Autodesk Inventor part; units mm, degrees
ref_plane "YZ Plane" through (0, 0, 0) normal (1, 0, 0) x (0, 1, 0)
ref_plane "XZ Plane" through (0, 0, 0) normal (0, 1, 0) x (-1, 0, 0)
ref_plane "XY Plane" through (0, 0, 0) normal (0, 0, 1) x (1, 0, 0)
sketch "Boceto1" plane through (0, 0, 0) normal (1, 0, 0) x (0, 1, 0)
  line L0 (0, 0) -> (0, -60)
  line L1 (0, -60) -> (10, -60)
  line L2 (10, -60) -> (10, -48)
  line L3 (10, -48) -> (35, -48)
  line L4 (35, -48) -> (35, -12)
  line L5 (35, -12) -> (10, -12)
  line L6 (10, -12) -> (10, 0)
  line L7 (10, 0) -> (0, 0)
  circle A0 centre (15, -30) radius 6
  dimension "d0" = 36
  dimension "d1" = 12
  dimension "d2" = 12
  dimension "d3" = 35
  dimension "d4" = 10
  dimension "d5" = 20
  dimension "d6" = 18
  dimension "d7" = 12
extrude "Extrusión1" add sketch "Boceto1" along normal blind 20
sketch "Boceto2" plane through (20, 0, 0) normal (1, 0, 0) x (0, 0, -1)
  circle A0 centre (30, 15) radius 6
  circle A1 centre (30, 15) radius 11
  point P0 (0, 0)
  dimension "d10" = 22
extrude "Extrusión2" cut sketch "Boceto2" against normal blind 7
sketch "Boceto3" plane through (0, 0, 0) normal (-1, 0, 0) x (0, 0, 1)
  circle A0 centre (-30, 15) radius 6
  circle A1 centre (-30, 15) radius 11
  point P0 (0, 0)
  dimension "d13" = 22
extrude "Extrusión3" cut sketch "Boceto3" against normal blind 7
sketch "Boceto4" plane through (0, 10, 0) normal (0, 1, 0) x (1, 0, 0)
  line L0 (20, 12) -> (20, 0)
  line L1 (0, 12) -> (0, 0)
  line L2 (20, 60) -> (20, 48)
  line L3 (0, 12) -> (20, 12)
  line L4 (0, 0) -> (20, 0)
  line L5 (0, 60) -> (20, 60)
  point P0 (10, 6)
  point P1 (10, 54)
  dimension "d16" = 20
  dimension "d17" = 10
  dimension "d18" = 10
  dimension "d19" = 12
  dimension "d20" = 6
  dimension "d21" = 6
hole "Agujero1" at (10, 10, -6) at (10, 10, -54) direction (0, -1, 0) diameter 5 end through all
fillet "Empalme1" radius 4 4 edges at (20, 5, 0) (20, 5, -60) (0, 5, -60) (0, 5, 0)
fillet "Empalme2" radius 2 2 edges at (10, 10, -12) (10, 10, -48)
fillet "Empalme3" radius 4 2 edges at (10, 35, -12) (10, 35, -48)
equation "\"d2\" = d1"
equation "\"d6\" = 0.5 * d0"
properties part number "Soporte_rueda_aluminio"
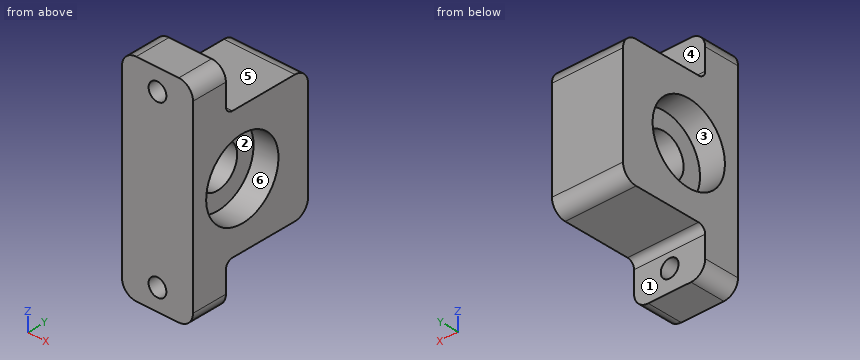
The model under review builds one solid part; all positions refer to its coordinate system, in mm. Face numbers are marked on the shaded views. A direction names the side the tool comes from. Give positions to 0.01 mm unless a question says otherwise; leave off trailing zeros. Write each loop counter-clockwise with the first axis right and the second up, starting at its lowest first coordinate (ties: lowest second). Pieces come first, ordered by that corner, then holes.
1. Wall thickness on L1, parallel to Z at x = 10, y = 3.5; L2, parallel to Z at x = 9.45, y = 15; L3, parallel to Y at x = 15.25, z = -30: over which ranges is each line inside the solid? List them lowest first.
2. Add section A-A, the plane x = 10. Write out the cut boundary in (y, z).
3. For P1, Ø11, axis at y = 14, z = -29, coming from the +X side; P2, Ø6, axis at x = 10, z = -54, coming from the +Y side; P3, Ø7, axis at y = 15, z = -30, coming from the +X side; P4, Ø8, axis at x = 11.5, y = 25, coming from the -Z side, all flat-tipped, find the tip position at first contact; note any pin that passes through.
4. Add section C-C, the plane y = 15. Write out the cut boundary in (x, z).
5. Draft analysis for pull direction Y (two halves, no side actions). For the marked faces 4, 5 and 6, state which applies: +Y half, -Y half, draft (parallel to the pull), parting line (faces both ways), or undercut.
6. Tool access review of the marked faces 1, 2 and 3: name each direction out of +Z, -Z, +X, -X, +Y, -Y from which nothing blocks a thin tool from reaching the whole face with its end or side.
7. Add section D-D, the plane x = 14.25. Write out the cut boundary in (y, z).
8. Add section B-B, the plane z = -30. Write out the cut boundary in (x, y).
Worked answers:
1. L1: z = -60 to -56.5, -51.5 to -8.5, -3.5 to 0
1. L2: z = -48 to -36, -24 to -12
1. L3: y = 0 to 4, 26 to 35
2. outline: (0, -60) - (10, -60) - (10, -56.5) - (0, -56.5) - close; (0, -51.5) - (10, -51.5) - (10, -50) arc R2 cw to (12, -48) - (31, -48) arc R4 ccw to (35, -44) - (35, -16) arc R4 ccw to (31, -12) - (12, -12) arc R2 cw to (10, -10) - (10, -8.5) - (0, -8.5) - close; (0, -3.5) - (10, -3.5) - (10, 0) - (0, 0) - close; hole circle Ø12 at (15, -30)
3. P1: stops at x = 13
3. P2: stops at y = 10
3. P3: passes through
3. P4: stops at z = -48
4. outline: (0, -48) - (20, -48) - (20, -41) - (13, -41) - (13, -36) - (7, -36) - (7, -41) - (0, -41) - close; (0, -19) - (7, -19) - (7, -24) - (13, -24) - (13, -19) - (20, -19) - (20, -12) - (0, -12) - close
5. face 4: +Y half
5. face 5: draft
5. face 6: undercut
6. face 1: -Z, +X, -X, +Y
6. face 2: +X
6. face 3: -X
7. outline: (0, -60) - (10, -60) - (10, -50) arc R2 cw to (12, -48) - (31, -48) arc R4 ccw to (35, -44) - (35, -16) arc R4 ccw to (31, -12) - (12, -12) arc R2 cw to (10, -10) - (10, 0) - (0, 0) - close; hole circle Ø22 at (15, -30)
8. outline: (0, 0) - (20, 0) - (20, 4) - (13, 4) - (13, 9) - (7, 9) - (7, 4) - (0, 4) - close; (0, 26) - (7, 26) - (7, 21) - (13, 21) - (13, 26) - (20, 26) - (20, 35) - (0, 35) - close
